Build history of the part. All positions in model axes, mm. Face numbers are marked on the shaded views. A direction names the side the tool comes from. Round coordinates to 2 decimals unless told otherwise and drop trailing zeros. Write each loop counter-clockwise with the first axis right and the second up, starting at its lowest first coordinate (ties: lowest second). Pieces come first, ordered by that corner, then holes.
1) Pull direction X, two halves, no side cores. Call the marked faces 3, 4 and 5: +X half, -X half, draft (parallel to the pull), parting line (faces both ways), or undercut.
2) Saw through at C-C (x = 0). State how many separate pieces and enclosed holes the cut face has, plus the area to 3 significant figures.
3) Which spindle directions (+Z, -Z, +X, -X, +Y, -Y) get a long thin tool onto all of the face, cutting with end or side? Do the marked faces 1 and 2. Say none if no direction does.
4) Flat gauge pins, fed straight in: pin 1 (2 mm diameter, centred on x = 17.5, z = 1.5, fed in from +Y); pin 2 (3 mm diameter, centred on x = 16, z = -11.5, fed in from -Y); pin 3 (4 mm diameter, centred on y = 1, z = 2.5, fed in from -X); pin 4 (4 mm diameter, centred on x = 0, z = 0, fed in from +Y). Where does each tip first touch, or does it go through?
5) Saw through at B-B (y = 11.25). Write the cut outline in (x, z) (3 decimals), plus the area to 3 significant figures.
6) Wall check: probe 1 along X at (y, z) = (-10.75, 9); probe 2 along X at (y, z) = (11.25, 1.5); probe 3 along Z at (x, y) = (-3.5, -5.5). Give the ranges that are in metal, low to high.
7) Saw through at A-A (y = 3.75). Write the cut outline in (x, z) (3 decimals).
from build123d import *

# Parameters (mm, degrees)
F5_DEPTH      = 25.401
F5_DEPTH_BACK = 25.4


with BuildPart() as f1:
    # F0 (on Right) → F1 (revolve)
    with BuildSketch(Plane.YZ):
        with BuildLine():
            Line((-12.7, 3.175), (12.7, 3.175))
            Line((12.7, 3.175), (12.7, 10.16))
            Line((12.7, 10.16), (10.16, 11.6264696837))
            Line((10.16, 11.6264696837), (10.16, 21.3935303163))
            Line((10.16, 21.3935303163), (12.7, 22.86))
            Line((12.7, 22.86), (12.7, 42.545))
            ThreePointArc((12.7, 42.545), (11.7700640303, 44.7900640303), (9.525, 45.72))
            Line((9.525, 45.72), (-9.525, 45.72))
            ThreePointArc((-9.525, 45.72), (-11.7700640303, 44.7900640303), (-12.7, 42.545))
            Line((-12.7, 42.545), (-12.7, 22.86))
            Line((-12.7, 22.86), (-10.16, 21.3935303163))
            Line((-10.16, 21.3935303163), (-10.16, 11.6264696837))
            Line((-10.16, 11.6264696837), (-12.7, 10.16))
            Line((-12.7, 10.16), (-12.7, 3.175))
        make_face()
    revolve(axis=Axis((0, -22.9387803917, 0), (0, -1, 0)))


with BuildPart() as f2_1:
    # F2: copy of F1
    add(f1.part)

    # F4 (on face) → F5 (cut, two sides)
    with BuildSketch(Plane.XZ.offset(12.7)) as f5_sk:
        with BuildLine():
            ThreePointArc((-5.0649481151, 32.6292307692), (0, 27.94), (5.0649481151, 32.6292307692))
            ThreePointArc((5.0649481151, 32.6292307692), (0, 33.02), (-5.0649481151, 32.6292307692))
        make_face()
        with BuildLine():
            ThreePointArc((-5.0649481151, 32.6292307692), (0, 33.02), (5.0649481151, 32.6292307692))
            ThreePointArc((5.0649481151, 32.6292307692), (5.076235634, 32.8244704939), (5.08, 33.02))
            ThreePointArc((5.08, 33.02), (-0.1955295061, 38.096235634), (-5.0649481151, 32.6292307692))
        make_face()
        with BuildLine():
            ThreePointArc((32.6292307692, -5.0649481151), (32.9221627479, -2.54), (33.02, 0))
            ThreePointArc((33.02, 0), (32.9221627479, 2.54), (32.6292307692, 5.0649481151))
            ThreePointArc((32.6292307692, 5.0649481151), (27.94, 0), (32.6292307692, -5.0649481151))
        make_face()
        with BuildLine():
            ThreePointArc((32.6292307692, 5.0649481151), (32.9221627479, 2.54), (33.02, 0))
            ThreePointArc((33.02, 0), (32.9221627479, -2.54), (32.6292307692, -5.0649481151))
            ThreePointArc((32.6292307692, -5.0649481151), (36.4711804001, -3.7277008794), (38.1, 0))
            ThreePointArc((38.1, 0), (36.4711804001, 3.7277008794), (32.6292307692, 5.0649481151))
        make_face()
        with BuildLine():
            ThreePointArc((-5.0649481151, -32.6292307692), (0, -33.02), (5.0649481151, -32.6292307692))
            ThreePointArc((5.0649481151, -32.6292307692), (0, -27.94), (-5.0649481151, -32.6292307692))
        make_face()
        with BuildLine():
            ThreePointArc((5.08, -33.02), (5.076235634, -32.8244704939), (5.0649481151, -32.6292307692))
            ThreePointArc((5.0649481151, -32.6292307692), (0, -33.02), (-5.0649481151, -32.6292307692))
            ThreePointArc((-5.0649481151, -32.6292307692), (-0.1955295061, -38.096235634), (5.08, -33.02))
        make_face()
        with BuildLine():
            ThreePointArc((-27.94, 0), (-29.2922991206, 3.4511804001), (-32.6292307692, 5.0649481151))
            ThreePointArc((-32.6292307692, 5.0649481151), (-33.02, 0), (-32.6292307692, -5.0649481151))
            ThreePointArc((-32.6292307692, -5.0649481151), (-29.2922991206, -3.4511804001), (-27.94, 0))
        make_face()
        with BuildLine():
            ThreePointArc((-32.6292307692, -5.0649481151), (-33.02, 0), (-32.6292307692, 5.0649481151))
            ThreePointArc((-32.6292307692, 5.0649481151), (-38.1, 0), (-32.6292307692, -5.0649481151))
        make_face()
    extrude(amount=-F5_DEPTH, mode=Mode.SUBTRACT)
    extrude(f5_sk.sketch, amount=F5_DEPTH_BACK, mode=Mode.SUBTRACT)


solid = f2_1.part
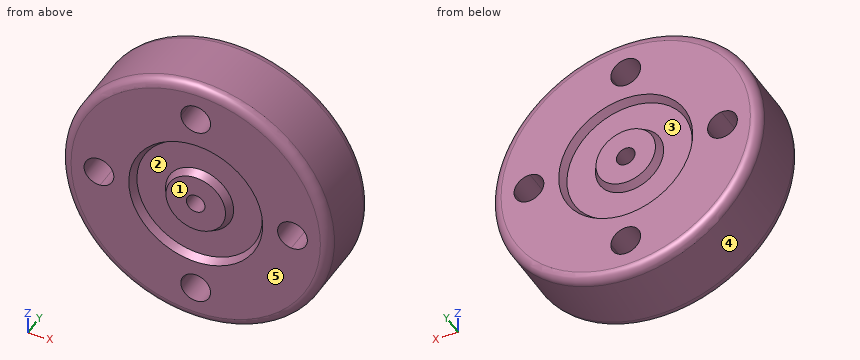
Evaluation:
1. face 3: undercut
1. face 4: parting line
1. face 5: draft
2. separate pieces: 4
2. enclosed holes: 0
2. area: 1,520 mm2
3. face 1: +Z, -Z, +X, -X, -Y
3. face 2: -Y
4. pin 1: stops at y = 10.16
4. pin 2: stops at y = -10.16
4. pin 3: stops at x = -45.72
4. pin 4: passes through
5. outline: circle Ø90.421 at (0, 0); circle Ø21.994 at (0, 0); hole circle Ø10.16 at (-33.02, 0); hole circle Ø44.046 at (0, 0); hole circle Ø10.16 at (0, -33.02); hole circle Ø10.16 at (0, 33.02); hole circle Ø6.35 at (0, 0); hole circle Ø10.16 at (33.02, 0)
5. area: 4,920 mm2
6. probe 1: x = -44.57 to -19.78, -6.81 to 6.81, 19.78 to 44.57
6. probe 2: x = -45.19 to -37.87, -28.17 to -21.97, -10.89 to -2.8, 2.8 to 10.89, 21.97 to 28.17, 37.87 to 45.19
6. probe 3: z = -45.59 to -36.7, -29.34 to 29.34, 36.7 to 45.59
7. outline: circle Ø91.44 at (0, 0); hole circle Ø10.16 at (-33.02, 0); hole circle Ø10.16 at (0, -33.02); hole circle Ø10.16 at (0, 33.02); hole circle Ø6.35 at (0, 0); hole circle Ø10.16 at (33.02, 0)
